Design review of the part shown in the three views and the two pictorial views. Dimensions are in mm from the part's minimum x, y and z. A direction names the side the tool comes from. Round coordinates to 2 decimals unless told otherwise and drop trailing zeros. Loops run counter-clockwise (first coordinate to the right, second up) from the corner with the lowest first, then second, coordinate; pieces in that order, holes last. Notation, with made-up numbers: (84, 57.25) -> (115, 57.25) arc R17 cw to (115, 78.25) -> close; hole circle Ø2 at (31.25, 51.5). An arc over 180 degrees is marked (long way). One line per question, with ' | ' between items. Start each with the question number.
1. For pin 1 Ø2 at (x, z) = (13.5, 4) entering from +Y; pin 2 Ø3 at (x, y) = (21.5, 6) entering from -Z; pin 3 Ø1 at (x, z) = (3, 4) entering from +Y, all flat-tipped, find the tip position at first contact; note any pin that passes through.
2. Wall thickness on line 1 along Z through (x, y) = (13.25, 6.25); line 2 along Y through (x, z) = (24.5, 9.25); line 3 along X through (y, z) = (3.75, 12) (1 decimal): over which ranges is each line inside the solid? List them lowest first.
3. For the marked faces 1, 2, 3 and 4, list the 3-axis set-ups (+Z, -Z, +X, -X, +Y, -Y) from which the entire face can be reached by the end or side of a thin tool; tool diameter is ignored.
4. Consider section D-D (x = 12.25). Write out the cut boundary in (y, z).
5. Consider section B-B (x = 25). Write out the cut boundary in (y, z).
6. Consider section A-A (z = 23.5). Write out the cut boundary in (x, y) (1 decimal), and give its area (3 significant figures).
7. Consider section C-C (y = 3.5). Write out the cut boundary in (x, z) (1 decimal).
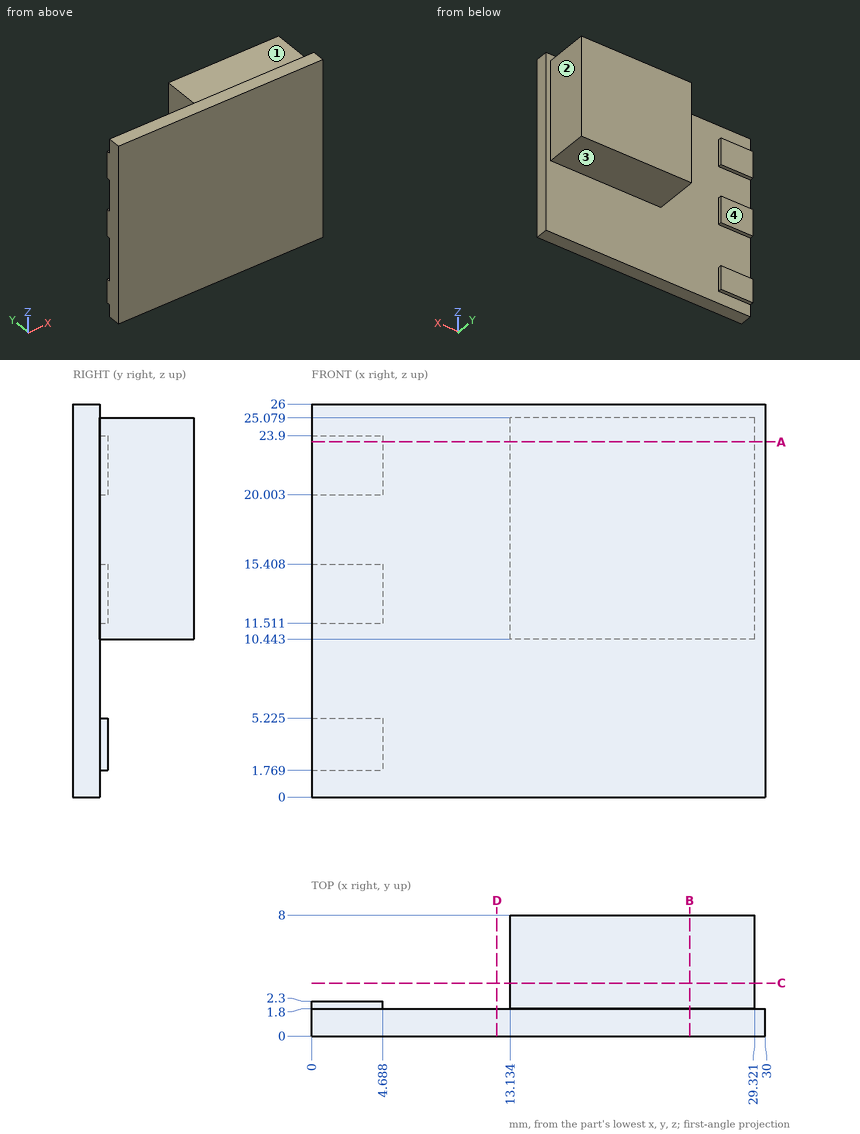
Answer block:
1) pin 1: stops at y = 1.8 | pin 2: stops at z = 10.44 | pin 3: stops at y = 2.3
2) line 1: z = 10.44 to 25.08 | line 2: y = 0 to 1.8 | line 3: x = 13.1 to 29.3
3) face 1: +Z, +X, -X, +Y | face 2: +Z, -Z, +X, +Y | face 3: -Z, +X, -X, +Y | face 4: +Z, -Z, -X, +Y
4) outline: (0, 0) -> (1.8, 0) -> (1.8, 26) -> (0, 26) -> close
5) outline: (0, 0) -> (1.8, 0) -> (1.8, 10.44) -> (8, 10.44) -> (8, 25.08) -> (1.8, 25.08) -> (1.8, 26) -> (0, 26) -> close
6) outline: (0, 0) -> (30, 0) -> (30, 1.8) -> (29.3, 1.8) -> (29.3, 8) -> (13.1, 8) -> (13.1, 1.8) -> (4.7, 1.8) -> (4.7, 2.3) -> (0, 2.3) -> close | area: 157 mm2
7) outline: (13.1, 10.4) -> (29.3, 10.4) -> (29.3, 25.1) -> (13.1, 25.1) -> close
